```python
from build123d import *

# Parameters (mm, degrees)
F0_R        = 15.875
F0_R_2      = 9.525
F1_DEPTH    = 25.4
F2_DEPTH    = 25.4
F3_DEPTH    = 12.7
F4_T1_DEPTH = 53.6792843218
F4_T3_DEPTH = 61.8868884968


# Not quite as in the source:
# - a fillet or chamfer that OpenCascade refuses, or shapes differently, is made with other operations: its cross-section is extruded or revolved along the edge and cut away or added


with BuildPart() as f1:
    # F0 (on Top) → F1 (new body)
    with BuildSketch(Plane.XY):
        with BuildLine():
            Line((10.035773719, 26.7546981082), (0, 28.575))
            ThreePointArc((0, 28.575), (-28.575, 0), (0, -28.575))
            Line((0, -28.575), (10.3516981132, -26.6340566038))
            ThreePointArc((10.3516981132, -26.6340566038), (23.5831549902, -16.135842888), (28.575, 0))
            ThreePointArc((28.575, 0), (23.4872610048, 16.2751096921), (10.035773719, 26.7546981082))
        make_face()
        Circle(F0_R, mode=Mode.SUBTRACT)
        with BuildLine():
            Line((54.1998407335, 18.7441613039), (10.035773719, 26.7546981082))
            ThreePointArc((10.035773719, 26.7546981082), (23.4872610048, 16.2751096921), (28.575, 0))
            ThreePointArc((28.575, 0), (23.5831549902, -16.135842888), (10.3516981132, -26.6340566038))
            Line((10.3516981132, -26.6340566038), (50.8, -19.05))
            ThreePointArc((50.8, -19.05), (31.8266137334, 1.7067845735), (54.1998407335, 18.7441613039))
        make_face()
        with BuildLine():
            ThreePointArc((69.85, 0), (65.4230890371, 12.2093311452), (54.1998407335, 18.7441613039))
            ThreePointArc((54.1998407335, 18.7441613039), (31.8266137334, 1.7067845735), (50.8, -19.05))
            ThreePointArc((50.8, -19.05), (64.2703841816, -13.4703841816), (69.85, 0))
        make_face()
        with Locations((50.8, 0)):
            Circle(F0_R_2, mode=Mode.SUBTRACT)
    extrude(amount=-F1_DEPTH)

    # F0 (on Top) → F2 (join)
    with BuildSketch(Plane.XY):
        with BuildLine():
            Line((10.035773719, 26.7546981082), (0, 28.575))
            ThreePointArc((0, 28.575), (-28.575, 0), (0, -28.575))
            Line((0, -28.575), (10.3516981132, -26.6340566038))
            ThreePointArc((10.3516981132, -26.6340566038), (23.5831549902, -16.135842888), (28.575, 0))
            ThreePointArc((28.575, 0), (23.4872610048, 16.2751096921), (10.035773719, 26.7546981082))
        make_face()
        Circle(F0_R, mode=Mode.SUBTRACT)
    extrude(amount=F2_DEPTH)

    # F0 (on Top) → F3 (cut)
    with BuildSketch(Plane.XY):
        with BuildLine():
            ThreePointArc((69.85, 0), (65.4230890371, 12.2093311452), (54.1998407335, 18.7441613039))
            ThreePointArc((54.1998407335, 18.7441613039), (31.8266137334, 1.7067845735), (50.8, -19.05))
            ThreePointArc((50.8, -19.05), (64.2703841816, -13.4703841816), (69.85, 0))
        make_face()
        with Locations((50.8, 0)):
            Circle(F0_R_2, mode=Mode.SUBTRACT)
    extrude(amount=-F3_DEPTH, mode=Mode.SUBTRACT)

    # F4: fillet of radius 5.08 on 3 edges, made by hand

    # F4_s2 → F4_t1 (cut)
    with BuildSketch(Plane.XY.offset(-12.7)):
        with BuildLine():
            ThreePointArc((34.6890404798, -22.07080491), (38.6066005598, -18.5769977583), (37.3417274119, -13.4824848951))
            ThreePointArc((37.3417274119, -13.4824848951), (43.5177900762, -17.6031792193), (50.8, -19.05))
            Line((50.8, -19.05), (34.6890404798, -22.07080491))
        make_face()
    extrude(amount=F4_T1_DEPTH, mode=Mode.SUBTRACT)

    # F4_s4 → F4_t3 (cut)
    with BuildSketch(Plane.XY.offset(-12.7)):
        with BuildLine():
            ThreePointArc((34.8409541818, 22.2555017147), (38.7915508617, 18.7449449078), (37.4849973575, 13.6239937108))
            ThreePointArc((37.4849973575, 13.6239937108), (45.2204267219, 18.2145782832), (54.1998407335, 18.7441613039))
            Line((54.1998407335, 18.7441613039), (34.8409541818, 22.2555017147))
        make_face()
    extrude(amount=F4_T3_DEPTH, mode=Mode.SUBTRACT)


solid = f1.part
```
Here's how the part is built. I have some questions about the finished solid (model axes, mm). A direction names the side the tool comes from. Give positions to 0.01 mm unless a question says otherwise; leave off trailing zeros. Write each loop counter-clockwise with the first axis right and the second up, starting at its lowest first coordinate (ties: lowest second). Pieces come first, ordered by that corner, then holes. Notation, with made-up numbers: (64.25, 86.5) -> (91.25, 86.5) arc R16 ccw to (91.25, 115.5) -> close; hole circle Ø8 at (2, 69). An arc over 180 degrees is marked (long way). Write each question's results on one line, items separated by ' | '.
Item 1: For pin 1 Ø1.5 at (x, z) = (26.5, -18.5) entering from -Y; pin 2 Ø3 at (y, z) = (10, 11) entering from -X; pin 3 Ø12 at (y, z) = (-5.5, 4.5) entering from -X (3 decimals), each with a flat end and sliding along its axis, tell me the tip position at first contact or that it passes through.
Output:
pin 1: stops at y = -23.75 | pin 2: stops at x = -27.28 | pin 3: stops at x = -28.575
Item 2: Suppose I cut it at B-B on x = 6.5. Write out the boundary of the cut face in (y, z), plus the area to 3 significant figures.
Output:
outline: (-27.36, -25.4) -> (-14.48, -25.4) -> (-14.48, 25.4) -> (-27.36, 25.4) -> close; (14.48, -25.4) -> (27.4, -25.4) -> (27.4, 25.4) -> (14.48, 25.4) -> close | area: 1,310 mm^2
Item 3: Suppose I cut it at A-A on y = 5. Write out the boundary of the cut face in (x, z), plus the area to 3 significant figures.
Output:
outline: (-28.13, -25.4) -> (-15.07, -25.4) -> (-15.07, 25.4) -> (-28.13, 25.4) -> close; (15.07, -25.4) -> (42.69, -25.4) -> (42.69, -12.7) -> (32.42, -12.7) -> (32.42, 0) -> (28.13, 0) -> (28.13, 25.4) -> (15.07, 25.4) -> close; (58.91, -25.4) -> (69.18, -25.4) -> (69.18, -12.7) -> (58.91, -12.7) -> close | area: 1,700 mm^2
Item 4: Suppose I cut it at D-D on y = -12. Write out the boundary of the cut face in (x, z), plus the area to 3 significant figures.
Output:
outline: (-25.93, -25.4) -> (-10.39, -25.4) -> (-10.39, 25.4) -> (-25.93, 25.4) -> close; (10.39, -25.4) -> (65.6, -25.4) -> (65.6, -12.7) -> (36, -12.7) -> (36, 0) -> (25.93, 0) -> (25.93, 25.4) -> (10.39, 25.4) -> close | area: 2,210 mm^2
Item 5: On a 3-axis mill with a long thin cutter (end or side, diameter ignored), from which of +Z, -Z, +X, -X, +Y, -Y can I reach the whole of each face in a straight line? I mean faces 1 (the face through (12, -12, 25.4)), 2 (the face through (31.753, 0.312, -6.261)). Say none if no direction works.
Output:
face 1: +Z, +X, -X, +Y, -Y | face 2: +Z, +X
Item 6: We'd pull the mould along Y, two halves only. Please class faces 3 (the face through (38.583, -18.651, -6.439)), 4 (the face through (42, 5, -12.7)), 5 (the face through (21.457, 24.683, -6)), 6 (the face through (69.734, -2.1, -18.961)): pulls with the +Y half, pulls with the -Y half, needs draft (parallel to the pull), parting line crosses it, or undercut.
Output:
face 3: undercut | face 4: undercut | face 5: pulls with the +Y half | face 6: parting line crosses it
Item 7: If I drill on L1, parallel to Y at x = 50.8, z = -18.5 (3 decimals); L2, parallel to Z at x = 54, y = -12.5; L3, parallel to X at y = 8, z = 5, over which ranges is the centre line in solid material (lowest first)?
Output:
L1: y = -19.05 to -9.525, 9.525 to 19.361 | L2: z = -25.4 to -12.7 | L3: x = -27.43 to -13.71, 13.71 to 27.43
